Study the drawing (mm; zero at the part's minimum x, y, z) and answer. A direction names the side the tool comes from. Round coordinates to 2 decimals unless told otherwise and drop trailing zeros. Write each loop counter-clockwise with the first axis right and the second up, starting at its lowest first coordinate (ties: lowest second). Pieces come first, ordered by that corner, then holes. Notation, with made-up numbers: (89.5, -19.5) -> (116.5, -19.5) arc R19 cw to (116.5, -13.5) -> close; hole circle Ø1 at (28, -23.5). An arc over 180 degrees is marked (long way). One line per question, with ' | ' between items. Start each with the question number.
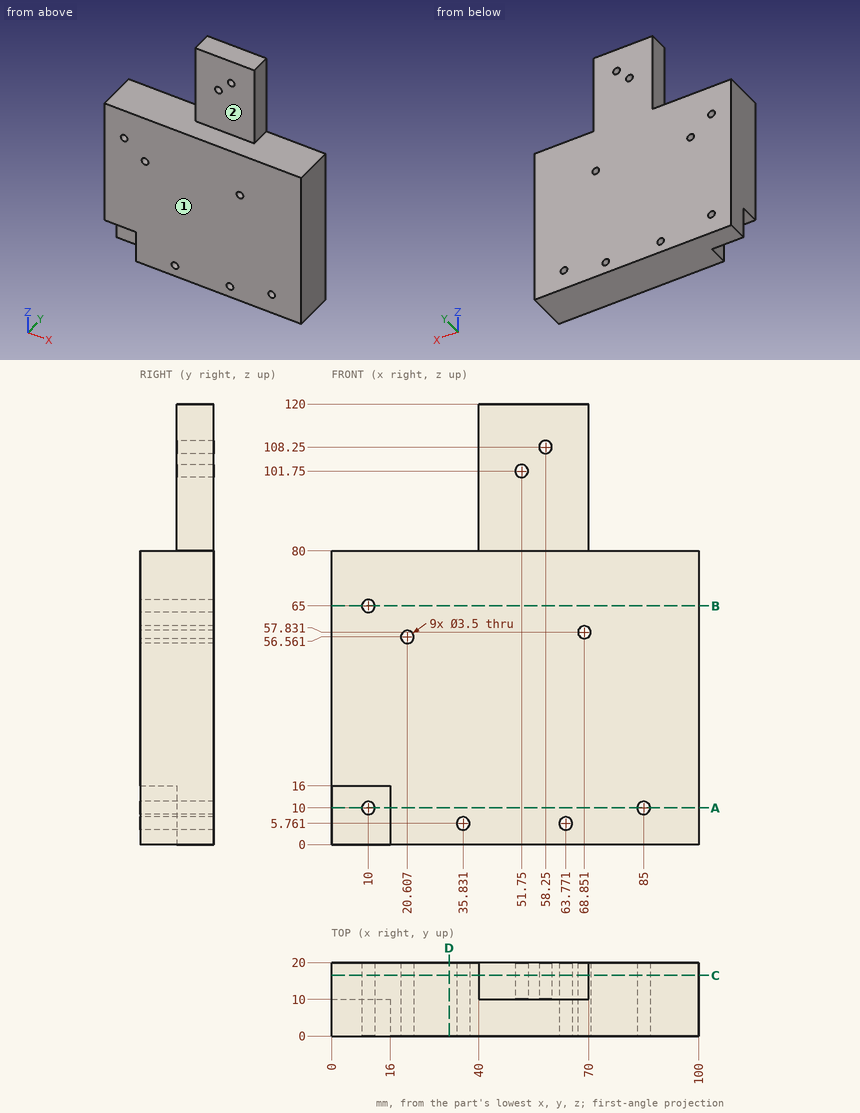
(1) For the marked faces 1 and 2, determine the directions among +Z, -Z, +X, -X, +Y, -Y from which every point of the face is accessible in a straight line to the end or side of a thin tool.
(2) A cutting plane is placed at B-B, the plane z = 65. Determine the outline of the cut face in (x, y).
(3) Given pin 1 Ø5 at (x, y) = (11, 7) entering from -Z; pin 2 Ø2 at (x, z) = (10, 10) entering from -Y; pin 3 Ø3 at (y, z) = (4, 10) entering from -X; pin 4 Ø8 at (y, z) = (14.5, 103.5) entering from +X, each flat-ended and moving along its own axis, determine where each tip first touches the part or whether it passes through.
(4) Consider L1, parallel to Z at x = 10, y = 17.5; L2, parallel to X at y = 4.75, z = 65; L3, parallel to Z at x = 87.5, y = 16.75. Determine where each line is inside the solid, lowest interval first.
(5) A cutting plane is placed at C-C, the plane y = 16.5. Count the separate pieces of the cut face and the enclosed holes in it, then the cut area to 3 significant figures.
(6) A cutting plane is placed at D-D, the plane x = 32. Determine the outline of the cut face in (y, z).
(7) A cutting plane is placed at A-A, the plane z = 10. Determine the outline of the cut face in (x, y).
Returned:
1) face 1: +Z, -Z, +X, -X, -Y | face 2: +Z, +X, -X, -Y
2) outline: (0, 0) -> (8.25, 0) -> (8.25, 20) -> (0, 20) -> close; (11.75, 0) -> (100, 0) -> (100, 20) -> (11.75, 20) -> close
3) pin 1: z = 16 | pin 2: through | pin 3: x = 16 | pin 4: x = 70
4) L1: 0 to 8.25, 11.75 to 63.25, 66.75 to 80 | L2: 0 to 8.25, 11.75 to 100 | L3: 0 to 80
5) separate pieces: 1 | enclosed holes: 9 | area: 9,110 mm2
6) outline: (0, 0) -> (20, 0) -> (20, 80) -> (0, 80) -> close
7) outline: (0, 10) -> (8.25, 10) -> (8.25, 20) -> (0, 20) -> close; (11.75, 10) -> (16, 10) -> (16, 0) -> (83.25, 0) -> (83.25, 20) -> (11.75, 20) -> close; (86.75, 0) -> (100, 0) -> (100, 20) -> (86.75, 20) -> close
